Design review of the part built by this model. Coordinates are the model's own, in mm. A direction names the side the tool comes from. Coordinates: 2 decimals unless noted, no trailing zeros. Loops run counter-clockwise (first coordinate to the right, second up) from the corner with the lowest first, then second, coordinate; pieces in that order, holes last. Notation, with made-up numbers: M -8.75,5.25 L 5.25,5.25 A21 cw 5.25,40.25 Z; hole C 67.25,-26.5 d10. An arc over 180 degrees is marked long. Put each result on its own line as item: value. Start each with the question number.
(1) For probe 1 along X at (y, z) = (-19.5, 29); probe 2 along Y at (x, z) = (-17, 42); probe 3 along Z at (x, y) = (-66, -12), list the stretches that pass through material, from the lowest coordinate up. Write a range as [from, to].
(2) Take a section at B-B, the plane z = 28.5. Give the boundary of the cut face in (x, y), then the cut area to 3 significant figures.
(3) Clearance check with flat-ended pins moving along their axes: pin 1 (1 mm diameter, centred on x = -63.5, y = -11.5, fed in from +Z); pin 2 (5 mm diameter, centred on x = -110.5, z = 40, fed in from -Y); pin 3 (6 mm diameter, centred on y = -15, z = 52, fed in from +X). State where each tip first meets the part, or that it passes through.
(4) For faces 1 (the cylindrical face through (-69.29, -39.85, 55.73)), 2 (the flat face through (-128, -20, 24)), list the 3-axis set-ups (+Z, -Z, +X, -X, +Y, -Y) from which the entire face can be reached by the end or side of a thin tool; tool diameter is ignored.
(5) The part is to be moulded in two halves that separate along X. For faces 3 (the cylindrical face through (-3.69, -19.47, 3.42)), 4 (the flat face through (0, -20, 31)), 5 (the flat face through (-67.901, -19.474, 56.067)), say which applies: +X half, -X half, draft (parallel to the pull), parting line (faces both ways), or undercut.
(6) Take a section at A-A, the plane y = -21. Give the boundary of the cut face in (x, z), then the cut area to 3 significant figures.
```python
from build123d import *

# Parameters (mm, degrees)
F1_DEPTH = 1
F2_DEPTH = 40
F3_R     = 0.5


with BuildPart() as f1:
    # F0 (on Front) → F1 (new body)
    with BuildSketch(Plane.XZ):
        with BuildLine():
            ThreePointArc((-16, 0), (-4.686292, 4.686292), (0, 16))
            Line((0, 16), (0, 45.592571))
            ThreePointArc((0, 45.592571), (-5.503554, 57.668358), (-18.228077, 61.436677))
            Line((-18.228077, 61.436677), (-118.531803, 47.331465))
            ThreePointArc((-118.531803, 47.331465), (-125.302103, 43.65495), (-128, 36.438643))
            Line((-128, 36.438643), (-128, 11))
            ThreePointArc((-128, 11), (-124.778175, 3.221825), (-117, 0))
            Line((-117, 0), (-16, 0))
        make_face()
    extrude(amount=F1_DEPTH)

    # F0 (on Front) → F2 (join)
    with BuildSketch(Plane.XZ):
        with BuildLine():
            ThreePointArc((-129.6, 11), (-125.909545, 2.090455), (-117, -1.6))
            Line((-117, -1.6), (-16, -1.6))
            ThreePointArc((-16, -1.6), (-3.554921, 3.554921), (1.6, 16))
            Line((1.6, 16), (1.6, 45.592571))
            ThreePointArc((1.6, 45.592571), (-4.453909, 58.875936), (-18.450885, 63.021087))
            Line((-18.450885, 63.021087), (-118.754611, 48.915876))
            ThreePointArc((-118.754611, 48.915876), (-126.509682, 44.704594), (-129.6, 36.438643))
            Line((-129.6, 36.438643), (-129.6, 11))
        make_face()
        with BuildLine():
            Line((0, 45.592571), (0, 16))
            ThreePointArc((0, 16), (-4.686292, 4.686292), (-16, 0))
            Line((-16, 0), (-117, 0))
            ThreePointArc((-117, 0), (-124.778175, 3.221825), (-128, 11))
            Line((-128, 11), (-128, 36.438643))
            ThreePointArc((-128, 36.438643), (-125.302103, 43.65495), (-118.531803, 47.331465))
            Line((-118.531803, 47.331465), (-18.228077, 61.436677))
            ThreePointArc((-18.228077, 61.436677), (-5.503554, 57.668358), (0, 45.592571))
        make_face(mode=Mode.SUBTRACT)
    extrude(amount=F2_DEPTH)

    # F3
    f3_edges = [f1.edges().sort_by_distance(p)[0] for p in [
        (-66.5, -40, -1.6),
        (-66.5, -40, 0),
    ]]
    fillet(f3_edges, radius=F3_R)


solid = f1.part
```
Computed values:
1. probe 1: x = [-129.6, -128], [0, 1.6]
1. probe 2: y = [-1, 0]
1. probe 3: z = [-1.6, 0], [54.72, 56.33]
2. outline: M -129.6,-39.5 A0.5 ccw -129.1,-40 L -128.5,-40 A0.5 ccw -128,-39.5 L -128,-1 L 0,-1 L 0,-39.5 A0.5 ccw 0.5,-40 L 1.1,-40 A0.5 ccw 1.6,-39.5 L 1.6,0 L -129.6,0 Z
2. area: 256 mm^2
3. pin 1: stops at z = 56.76
3. pin 2: stops at y = -1
3. pin 3: stops at x = 1.27
4. face 1: +Z, -X, -Y
4. face 2: -Y
5. face 3: +X half
5. face 4: undercut
5. face 5: -X half
6. outline: M -129.6,11 A12.6 ccw -117,-1.6 L -16,-1.6 A17.6 ccw 1.6,16 L 1.6,45.59 A17.6 ccw -18.45,63.02 L -118.75,48.92 A12.6 ccw -129.6,36.44 Z; hole M -128,11 A11 ccw -117,0 L -16,0 A16 ccw 0,16 L 0,45.59 A16 ccw -18.23,61.44 L -118.53,47.33 A11 ccw -128,36.44 Z
6. area: 557 mm^2
